The model under review builds one solid part; all positions refer to its coordinate system, in mm. Face numbers are marked on the shaded views. A direction names the side the tool comes from. Round coordinates to 2 decimals unless told otherwise and drop trailing zeros. Write each loop counter-clockwise with the first axis right and the second up, starting at its lowest first coordinate (ties: lowest second). Pieces come first, ordered by that corner, then holes. Notation, with made-up numbers: M 18.25,-9 L 73.25,-9 A22 ccw 73.25,11 Z; hole C -39,24.5 d10. An arc over 180 degrees is marked long. One line per item, written item: value. Start each with the question number.
1) Mouldability with a two-part tool opening along Y and no side actions: class the marked faces 1 and 2 as +Y half, -Y half, draft (parallel to the pull), parting line (faces both ways), or undercut.
2) Take a section at B-B, the plane z = -10. Write out the cut boundary in (x, y).
3) Tool access review of the marked faces 3, 4, 5 and 6: name each direction out of +Z, -Z, +X, -X, +Y, -Y from which nothing blocks a thin tool from reaching the whole face with its end or side.
4) Take a section at A-A, the plane y = 0. Write out the cut boundary in (x, z).
5) Take a section at D-D, the plane x = 1. State how many separate pieces and enclosed holes the cut face has, and give its area (3 significant figures).
6) Take a section at C-C, the plane y = 58. Write out the cut boundary in (x, z).
7) Wall thickness on probe 1 along Y at (x, z) = (-1.5, -4); probe 2 along X at (y, z) = (-8.5, 5.25); probe 3 along Y at (x, z) = (13, -26): over which ranges is each line inside the solid? List them lowest first.
8) For P1, Ø3, axis at x = -6.5, y = 22, coming from the -Z side; P2, Ø1.5, axis at y = -26.5, z = 3.5, coming from the -X side; P3, Ø4.5, axis at x = 8.49, y = 8.49, coming from the +Z side; P4, Ø7.5, axis at x = -8.5, y = -8.5, coming from the -Z side, all flat-tipped, find the tip position at first contact; note any pin that passes through.
Autodesk Fusion 360 part; units mm, degrees
sketch "Sketch1" plane through (0, 0, 0) normal (0, 0, 1) x (1, 0, 0)
  line L0 (-20, -55) -> (20, -55)
  line L1 (20, -55) -> (20, 55)
  line L2 (20, 55) -> (-20, 55)
  line L3 (-20, 55) -> (-20, -55)
  circle A0 centre (0, 0) radius 23
  circle A1 centre (0, 55) radius 20
  circle A2 centre (0, -55) radius 18
extrude "Extrude1" add sketch "Sketch1" along normal blind 5
sketch "Sketch2" plane through (0, 0, 0) normal (0, 0, 1) x (1, 0, 0)
  circle A0 centre (0, 0) radius 17
extrude "Extrude2" add sketch "Sketch2" along normal blind 14
ref_plane "WorkPlane2" through (0, 0, -38) normal (0, 0, 1) x (1, 0, 0)
sketch "Sketch4" plane through (0, 0, -38) normal (0, 0, 1) x (1, 0, 0)
  circle A0 centre (0, 55) radius 20
extrude "Extrude4" add sketch "Sketch4" along normal blind 46
ref_plane "WorkPlane3" through (0, 0, -6) normal (0, 0, 1) x (1, 0, 0)
sketch "Sketch5" plane through (0, 0, -6) normal (0, 0, 1) x (1, 0, 0)
  line L0 (-14.55, -8) -> (14.55, -8)
  line L1 (14.55, -8) -> (14.55, 8)
  line L2 (14.55, 8) -> (-14.55, 8)
  line L3 (-14.55, 8) -> (-14.55, -8)
extrude "Extrude5" add sketch "Sketch5" along normal blind 7
ref_plane "WorkPlane4" through (0, 0, -36) normal (0, 0, 1) x (1, 0, 0)
sketch "Sketch6" plane through (0, 0, -36) normal (0, 0, 1) x (1, 0, 0)
  line L0 (-12.15, -8) -> (-14.55, -8)
  line L1 (-14.55, -8) -> (-14.55, 8)
  line L2 (-14.55, 8) -> (-12.15, 8)
  line L3 (-12.15, 8) -> (-12.15, -8)
  line L4 (12.15, -8) -> (14.55, -8)
  line L5 (14.55, -8) -> (14.55, 8)
  line L6 (14.55, 8) -> (12.15, 8)
  line L7 (12.15, 8) -> (12.15, -8)
extrude "Extrude6" add sketch "Sketch6" along normal blind 31
ref_plane "WorkPlane5" through (0, 0, -36) normal (0, 0, 1) x (1, 0, 0)
sketch "Sketch7" plane through (0, 0, -36) normal (0, 0, 1) x (1, 0, 0)
  line L0 (-10.55, -8) -> (-14.55, -8)
  line L1 (-14.55, -8) -> (-14.55, 8)
  line L2 (-14.55, 8) -> (-10.55, 8)
  line L3 (-10.55, 8) -> (-10.55, -8)
  line L4 (10.55, -8) -> (14.55, -8)
  line L5 (14.55, -8) -> (14.55, 8)
  line L6 (14.55, 8) -> (10.55, 8)
  line L7 (10.55, 8) -> (10.55, -8)
extrude "Extrude7" add sketch "Sketch7" along normal blind 2.5
ref_plane "WorkPlane6" through (0, 0, -7) normal (0, 0, 1) x (1, 0, 0)
sketch "Sketch8" plane through (0, 0, -7) normal (0, 0, 1) x (1, 0, 0)
  circle A0 centre (8.4853, 8.4853) radius 1.7
  circle A1 centre (-8.4853, 8.4853) radius 1.7
  circle A2 centre (-8.4853, -8.4853) radius 1.7
  circle A3 centre (8.4853, -8.4853) radius 1.7
extrude "Extrude8" cut sketch "Sketch8" along normal blind 22
ref_plane "WorkPlane7" through (0, 0, -7) normal (0, 0, 1) x (1, 0, 0)
sketch "Sketch9" plane through (0, 0, -7) normal (0, 0, 1) x (1, 0, 0)
  circle A0 centre (0, 0) radius 6
extrude "Extrude9" cut sketch "Sketch9" along normal blind 22
ref_plane "WorkPlane8" through (0, 0, -21) normal (0, 0, 1) x (1, 0, 0)
sketch "Sketch10" plane through (0, 0, -21) normal (0, 0, 1) x (1, 0, 0)
  circle A0 centre (0, -55) radius 6
extrude "Extrude10" cut sketch "Sketch10" along normal blind 30
ref_plane "WorkPlane9" through (0, 0, -39) normal (0, 0, 1) x (1, 0, 0)
sketch "Sketch11" plane through (0, 0, -39) normal (0, 0, 1) x (1, 0, 0)
  circle A0 centre (0, 55) radius 8.4
extrude "Extrude11" cut sketch "Sketch11" along normal blind 48
ref_plane "WorkPlane10" through (0, 0, -3.5) normal (0, 0, 1) x (1, 0, 0)
sketch "Sketch12" plane through (0, 0, -3.5) normal (0, 0, 1) x (1, 0, 0)
  circle A0 centre (0, 55) radius 16
extrude "Extrude12" cut sketch "Sketch12" along normal blind 12.5
ref_plane "WorkPlane11" through (0, 0, -39) normal (0, 0, 1) x (1, 0, 0)
sketch "Sketch13" plane through (0, 0, -39) normal (0, 0, 1) x (1, 0, 0)
  line L0 (0, 54.4) -> (40, 54.4)
  line L1 (40, 54.4) -> (40, 55.6)
  line L2 (40, 55.6) -> (0, 55.6)
  line L3 (0, 55.6) -> (0, 54.4)
extrude "Extrude13" cut sketch "Sketch13" along normal blind 36.5
ref_plane "WorkPlane12" through (0, 55, 0) normal (0, 1, 0) x (0, 0, 1)
sketch "Sketch14" plane through (0, 55, 0) normal (0, 1, 0) x (1, 0, 0)
  circle A0 centre (14, 21) radius 1.6
extrude "Extrude14" cut sketch "Sketch14" along normal mid plane 50
sketch "CupBossHoles" plane through (0, 0, -21) normal (0, 0, 1) x (1, 0, 0)
  circle A0 centre (-8.5, -63.5) radius 1.7
  circle A1 centre (-8.5, -46.5) radius 1.7
  circle A2 centre (8.5, -63.5) radius 1.7
  circle A3 centre (8.5, -46.5) radius 1.7
extrude "CupBossHolesCut" cut sketch "CupBossHoles" along normal blind 30
sketch "CupScrewCounterbores" plane through (0, 0, 0) normal (0, 0, 1) x (1, 0, 0)
  circle A0 centre (-8.5, -63.5) radius 3.25
  circle A1 centre (-8.5, -46.5) radius 3.25
  circle A2 centre (8.5, -63.5) radius 3.25
  circle A3 centre (8.5, -46.5) radius 3.25
extrude "CupScrewCounterboresCut" cut sketch "CupScrewCounterbores" along normal through all from surface at 2
sketch "MainScrewCounterbores" plane through (0, 0, -7) normal (0, 0, 1) x (1, 0, 0)
  circle A0 centre (-8.5, -8.5) radius 3.25
  circle A1 centre (-8.5, 8.5) radius 3.25
  circle A2 centre (8.5, -8.5) radius 3.25
  circle A3 centre (8.5, 8.5) radius 3.25
extrude "MainScrewCounterboresCut" cut sketch "MainScrewCounterbores" along normal blind 19
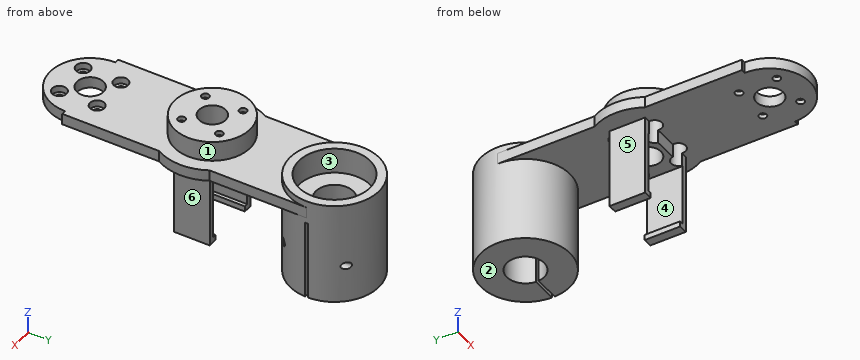
Checked values:
1. face 1: undercut
1. face 2: draft
2. outline: M -14.55,-8 L -12.15,-8 L -12.15,8 L -14.55,8 Z; M 8.38,54.4 A8.4 cw long 8.38,55.6 L 19.99,55.6 A20 ccw long 19.99,54.4 Z; M 12.15,-8 L 14.55,-8 L 14.55,8 L 12.15,8 Z
3. face 3: +Z
3. face 4: -Y
3. face 5: -Z, -X, -Y
3. face 6: -Z, +X, -Y
4. outline: M -23,0 L -14.55,0 L -14.55,-36 L -10.55,-36 L -10.55,-33.5 L -12.15,-33.5 L -12.15,-6 L -6,-6 L -6,14 L -17,14 L -17,5 L -23,5 Z; M 6,-6 L 12.15,-6 L 12.15,-33.5 L 10.55,-33.5 L 10.55,-36 L 14.55,-36 L 14.55,0 L 23,0 L 23,5 L 17,5 L 17,14 L 6,14 Z
5. separate pieces: 4
5. enclosed holes: 0
5. area: 1,540 mm2
6. outline: M -19.77,-38 L -7.85,-38 L -7.85,-3.5 L -15.72,-3.5 L -15.72,8 L -19.77,8 Z; M 7.85,-38 L 19.77,-38 L 19.77,8 L 15.72,8 L 15.72,-3.5 L 7.85,-3.5 Z; hole C 14,-21 d3.2
7. probe 1: y = -8 to -5.81, 5.81 to 8, 35.06 to 46.74, 63.26 to 74.94
7. probe 2: x = -14.72 to -11.75, -5.25 to 5.25, 11.75 to 14.72
7. probe 3: y = -8 to 8, 39.8 to 54.4, 55.6 to 70.2
8. P1: stops at z = 0
8. P2: stops at x = -20
8. P3: stops at z = 14
8. P4: stops at z = -36
